Build history of the part. All positions in model axes, mm. Face numbers are marked on the shaded views. Give positions to 0.01 mm unless a question says otherwise; leave off trailing zeros. Write each loop counter-clockwise with the first axis right and the second up, starting at its lowest first coordinate (ties: lowest second). Pieces come first, ordered by that corner, then holes. Notation, with made-up numbers: (87, -8) -> (128, -8) arc R26 ccw to (128, 15) -> close; hole circle Ø8 at (82.5, -30.75). An arc over 180 degrees is marked (long way). Put each result on its own line as item: value. Start each with the question number.
Item 1: Slice it at D-D, the plane y = -38. List the corners of the cut face in (x, z).
Item 2: Flat gauge pins, fed straight in: pin 1 Ø6 at (x, z) = (40.5, 19) entering from +Y; pin 2 Ø10 at (x, z) = (52.5, 36.5) entering from -Y; pin 3 Ø1.5 at (x, y) = (41.5, -7) entering from -Z; pin 4 Ø12 at (y, z) = (-11.5, 19.5) entering from -X. Where does each tip first touch, or does it go through?
Item 3: Slice it at B-B, the plane z = 0. List the corners of the cut face in (x, y).
Item 4: Slice it at A-A, the plane y = 0. List the corners of the cut face in (x, z), plus the area to 3 significant figures.
Item 5: Drill centre lines: line 1 along X through (y, z) = (-8, 41); line 2 along Y through (x, z) = (97.5, 0); line 3 along Z through (x, y) = (73, 0). Where is each one in solid material? Low to high.
Item 6: Two-plate mould, pull along X, no slides. Class the marked faces 1, 2 and 3: pulls with the +X half, pulls with the -X half, needs draft (parallel to the pull), parting line crosses it, or undercut.
Item 7: Slice it at C-C, the plane y = -20.5. List the corners of the cut face in (x, z), plus the area to 3 significant figures.
```python
from build123d import *

# Parameters (mm, degrees)
SKETCH2_R                   = 30
CUT_EXTRUDE1_DEPTH          = 143.788304843
BOSS_EXTRUDE1_REACH         = 164.242
BOSS_EXTRUDE1_END_RADIUS    = 40
SKETCH3_R                   = 8
M10X1_0_TAPPED_HOLE1_REACH  = 164.242
M10X1_0_TAPPED_HOLE1_BORE_R = 4.5
CUT_EXTRUDE2_DEPTH          = 143.788304931
CUT_EXTRUDE2_DEPTH_BACK     = 143.788304931


with BuildPart() as part:
    # Sketch1 → Revolve1 (revolve)
    with BuildSketch(Plane.XY, mode=Mode.PRIVATE) as revolve1_sk:
        Polygon((0, 0), (0, 47.5), (13, 47.5), (13, 40), (113, 40), (113, 47.5), (126, 47.5), (126, 0), align=None)
    revolve(revolve1_sk.sketch.rotate(Axis((126, 0, 0), (-1, 0, 0)), 90), axis=Axis((126, 0, 0), (-1, 0, 0)))

    # Sketch2 → Cut-Extrude1 (cut, through all)
    with BuildSketch(Plane(origin=(126, 0, 0), x_dir=(0, 0, -1), z_dir=(1, 0, 0))):
        Circle(SKETCH2_R)
    extrude(amount=-CUT_EXTRUDE1_DEPTH, mode=Mode.SUBTRACT)

    # Boss-Extrude1: up to this cylinder (the profile starts outside it)
    boss_extrude1_end = Plane(origin=(63, 0, 0), z_dir=(1, 0, 0)) * Cylinder(BOSS_EXTRUDE1_END_RADIUS, 409.484, mode=Mode.PRIVATE)
    # Sketch3 → Boss-Extrude1 (add, up to the surface)
    with BuildSketch(Plane(origin=(0, 43, 0), x_dir=(1, 0, 0), z_dir=(0, 1, 0)), mode=Mode.PRIVATE) as boss_extrude1_sk1:
        with Locations(Location((63, 0, 0), (0, 0, 270))):
            Circle(SKETCH3_R)
    boss_extrude1_tool1 = extrude(boss_extrude1_sk1.sketch, amount=-BOSS_EXTRUDE1_REACH, mode=Mode.PRIVATE) - boss_extrude1_end
    add(boss_extrude1_tool1.solids().sort_by_distance((63, 43, 0))[0])

    # M10x1.0 Tapped Hole1 bore → M10x1.0 Tapped Hole1 (cut, up to next)
    with BuildSketch(Plane(origin=(0, 43, 0), x_dir=(1, 0, 0), z_dir=(0, 1, 0)), mode=Mode.PRIVATE) as m10x1_0_tapped_hole1_sk1:
        with Locations((63, 0)):
            Circle(M10X1_0_TAPPED_HOLE1_BORE_R)
    m10x1_0_tapped_hole1_tool1 = extrude(m10x1_0_tapped_hole1_sk1.sketch, amount=-M10X1_0_TAPPED_HOLE1_REACH, mode=Mode.PRIVATE) & part.part
    add(m10x1_0_tapped_hole1_tool1.solids().sort_by_distance((63, 43, 0))[0], mode=Mode.SUBTRACT)

    # Sketch6 → Cut-Extrude2 (cut, two sides: drawn at the far end of the back side and taken through both)
    with BuildSketch(Plane(origin=(126, 0, 0), x_dir=(0, 0, -1), z_dir=(1, 0, 0)).offset(-CUT_EXTRUDE2_DEPTH_BACK)):
        Polygon((-315.109988933, 5), (-62.08548164, 5), (59.692601542, 5), (312.717108835, 5), (312.717108835, 511.049014586), (-315.109988933, 511.049014586), align=None)
    extrude(amount=CUT_EXTRUDE2_DEPTH + CUT_EXTRUDE2_DEPTH_BACK, mode=Mode.SUBTRACT)


solid = part.part
```
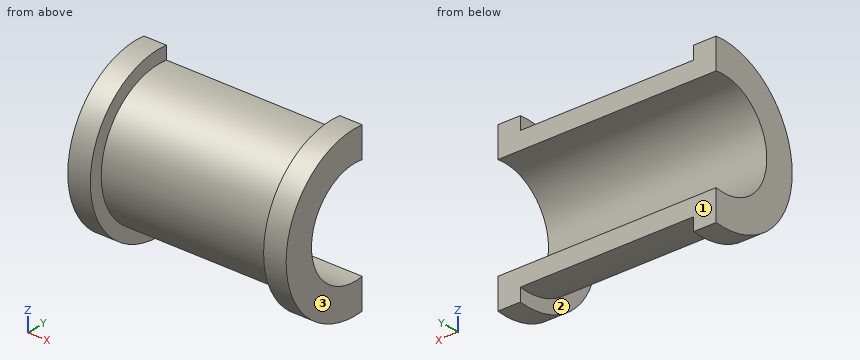
Values follow:
1. outline: (0, -28.5) -> (13, -28.5) -> (13, -12.49) -> (113, -12.49) -> (113, -28.5) -> (126, -28.5) -> (126, 28.5) -> (113, 28.5) -> (113, 12.49) -> (13, 12.49) -> (13, 28.5) -> (0, 28.5) -> close
2. pin 1: y = -20.4
2. pin 2: y = -24.65
2. pin 3: z = -39.51
2. pin 4: through
3. outline: (0, -47.5) -> (13, -47.5) -> (13, -40) -> (113, -40) -> (113, -47.5) -> (126, -47.5) -> (126, -30) -> (0, -30) -> close
4. outline: (0, -47.5) -> (13, -47.5) -> (13, -40) -> (113, -40) -> (113, -47.5) -> (126, -47.5) -> (126, -30) -> (0, -30) -> close; (0, 30) -> (126, 30) -> (126, 47.5) -> (113, 47.5) -> (113, 40) -> (13, 40) -> (13, 47.5) -> (0, 47.5) -> close
4. area: 2,910 mm2
5. line 1: 0 to 13, 113 to 126
5. line 2: -40 to -30
5. line 3: -40 to -30, 30 to 40
6. face 1: needs draft
6. face 2: undercut
6. face 3: pulls with the +X half
7. outline: (0, -42.85) -> (13, -42.85) -> (13, -34.35) -> (113, -34.35) -> (113, -42.85) -> (126, -42.85) -> (126, -21.9) -> (0, -21.9) -> close; (0, 21.9) -> (126, 21.9) -> (126, 42.85) -> (113, 42.85) -> (113, 34.35) -> (13, 34.35) -> (13, 42.85) -> (0, 42.85) -> close
7. area: 3,580 mm2
